Verification items for the finished model (mm, model axes). Face numbers are marked on the shaded views. A direction names the side the tool comes from. Coordinates: 2 decimals unless noted, no trailing zeros. Order: outer loops, then holes, each group sorted by start corner. A loop starts at its lowest first (then second) coordinate and runs counter-clockwise, first axis right, second up.
Q1. Depth check by flat-ended pin: P1, Ø4, axis at x = 37, z = 5, coming from the +Y side; P2, Ø3.5, axis at y = 47.5, z = 4, coming from the -X side; P3, Ø2.5, axis at y = 17, z = 2, coming from the +X side. Enter the tip coordinate at first touch or a pass-through.
Q2. Set-up check for the marked faces 1, 2 and 3: record each of +Z, -Z, +X, -X, +Y, -Y from which the full face is reachable in a straight line by a thin tool's end or side.
Q3. Cross-section at C-C, the plane z = 4. Record the boundary of the cut face in (x, y), and give its area (3 significant figures).
Q4. Cross-section at A-A, the plane x = 66.5. Record the boundary of the cut face in (y, z), and give its area (3 significant figures).
Q5. Thickness scan on line 1 (Z direction, x = 66.5, y = 3.65); line 2 (Y direction, x = 41, z = 1.5); line 3 (X direction, y = 38, z = 1). Record the ranges inside material, lowest first.
Q6. Cross-section at D-D, the plane y = 29. Record the boundary of the cut face in (x, z).
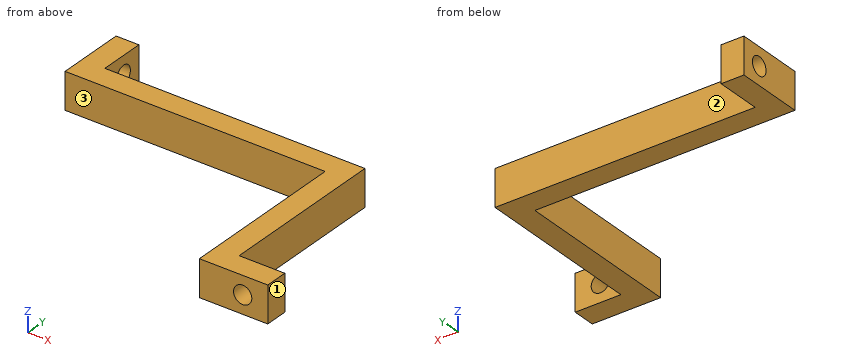
Autodesk Inventor part; units mm, degrees
ref_plane "YZ Plane" through (0, 0, 0) normal (1, 0, 0) x (0, 1, 0)
ref_plane "XZ Plane" through (0, 0, 0) normal (0, 1, 0) x (-1, 0, 0)
ref_plane "XY Plane" through (0, 0, 0) normal (0, 0, 1) x (1, 0, 0)
sketch "Sketch1" plane through (0, 0, 0) normal (0, 0, 1) x (1, 0, 0)
  line L0 (0, 37) -> (0, 52)
  line L1 (0, 52) -> (5, 52)
  line L2 (5, 52) -> (5, 42)
  line L3 (5, 42) -> (62, 42)
  line L4 (62, 42) -> (62, 5)
  line L5 (62, 5) -> (72, 5)
  line L6 (72, 5) -> (72, 0)
  line L7 (72, 0) -> (57, 0)
  line L8 (57, 0) -> (57, 37)
  line L9 (57, 37) -> (0, 37)
  point P0 (0, 0)
  dimension "d0" = 37
  dimension "d1" = 57
  dimension "d2" = 5
  dimension "d3" = 5
  dimension "d4" = 5
  dimension "d5" = 5
  dimension "d6" = 15
  dimension "d7" = 15
extrude "Extrusion1" add sketch "Sketch1" along normal blind 8
sketch "Sketch2" plane through (0, 37, 0) normal (-1, 0, 0) x (0, 0, 1)
  circle A0 centre (4, 10.5) radius 2
  line L0 (0, 15) -> (8, 15)
  point P0 (0, -37)
  point P1 (4, 15)
  dimension "d10" = 4
  dimension "d11" = 4.5
extrude "Extrusion2" cut sketch "Sketch2" against normal up to next
sketch "Sketch3" plane through (57, 0, 0) normal (0, -1, 0) x (1, 0, 0)
  circle A0 centre (9.5, 4) radius 2
  line L0 (15, 0) -> (15, 8)
  point P0 (-57, 0)
  point P1 (15, 4)
  dimension "d14" = 4
  dimension "d15" = 5.5
extrude "Extrusion3" cut sketch "Sketch3" against normal up to next
equation "\"d3\" = d2"
equation "\"d4\" = d2"
equation "\"d5\" = d2"
properties material "ABS Plastic"
Check values:
1. P1: stops at y = 42
1. P2: passes through
1. P3: stops at x = 62
2. face 1: +Z, -Z, +X, +Y, -Y
2. face 2: +Z, -Z, +X, +Y
2. face 3: +Z, -Z, -X, -Y
3. outline: (0, 37) - (57, 37) - (57, 0) - (64.5, 0) - (64.5, 5) - (62, 5) - (62, 42) - (5, 42) - (5, 45.5) - (0, 45.5) - close; (0, 49.5) - (5, 49.5) - (5, 52) - (0, 52) - close; (68.5, 0) - (72, 0) - (72, 5) - (68.5, 5) - close
3. area: 555 mm2
4. outline: (0, 0) - (5, 0) - (5, 2) - (0, 2) - close; (0, 6) - (5, 6) - (5, 8) - (0, 8) - close
4. area: 20.0 mm2
5. line 1: z = 0 to 2, 6 to 8
5. line 2: y = 37 to 42
5. line 3: x = 0 to 62
6. outline: (57, 0) - (62, 0) - (62, 8) - (57, 8) - close
